Geometry check sheet. Reference: the model listing, model coordinates, mm. A direction names the side the tool comes from. Coordinates: 2 decimals unless noted, no trailing zeros. Order: outer loops, then holes, each group sorted by start corner. A loop starts at its lowest first (then second) coordinate and runs counter-clockwise, first axis right, second up. Notation, with made-up numbers: M 38.5,89.5 L 95.5,89.5 A16 ccw 95.5,106.5 Z; hole C 44,57.5 d5. An arc over 180 degrees is marked long. One line per item, written item: value. Start each with the question number.
1) Draft check along Y on faces 1 (the flat face through (-51, 76.2, 13)), 2 (the flat face through (-38.1, 0, 13)), 3 (the flat face through (-2, 14, 0)), 4 (the flat face through (36.512, 0, 13)). Enter one of: pulls with the +Y half, pulls with the -Y half, needs draft (parallel to the pull), parting line crosses it, or undercut.
2) Access from +Z, -Z, +X, -X, +Y, -Y to the whole of each face (thin tool, end or side, straight path). Record for faces 5 (the flat face through (141.288, 17, 13)), 6 (the flat face through (-141.288, 18, 13)), 7 (the flat face through (141.288, -18, 13)), 8 (the flat face through (38.1, 0, 13)).
3) Go/stop test with flat-tipped pins: P1, Ø8, axis at y = -14, z = 18, coming from the +X side; P2, Ø8, axis at y = 16, z = 17, coming from the -X side; P3, Ø2, axis at x = 81.5, z = 6.5, coming from the -Y side. Record where each tip stops, or that it passes through.
4) Thickness scan on L1, parallel to X at y = -6, z = 11.25 (1 decimal); L2, parallel to Y at x = 88, z = 10.5; L3, parallel to X at y = 62.5, z = 16.5. Record the ranges inside material, lowest first. Write a range as from..to.
5) Sectioned sample at B-B, the plane x = -116. Enter the section's corners in (y, z), then the cut area to 3 significant figures.
6) Sectioned sample at C-C, the plane y = 40. Enter the section's corners in (x, z).
7) Sectioned sample at A-A, the plane z = 13.75. State how many separate pieces and enclosed holes the cut face has, then the cut area to 3 significant figures.
```python
from build123d import *

# Parameters (mm, degrees)
F0_W     = 25.4
F0_H     = 50.8
F0_W_2   = 76.2
F0_W_3   = 1.5875
F0_H_2   = 19.05
F1_DEPTH = 25.4


with BuildPart() as f1:
    # F0 (on Top) → F1 (new body)
    with BuildSketch(Plane.XY):
        Polygon((63.5, 25.4), (38.1, 25.4), (38.1, 9.525), (38.1, -9.525), (38.1, -25.4), (63.5, -25.4), (88.9, -25.4), (88.9, 25.4), align=None)
        with Locations((50.8, 50.8)):
            Rectangle(F0_W, F0_H)
        with Locations((0, 50.8)):
            Rectangle(F0_W_2, F0_H)
        Polygon((-38.1, 9.525), (-38.1, 25.4), (-63.5, 25.4), (-88.9, 25.4), (-88.9, -25.4), (-63.5, -25.4), (-38.1, -25.4), (-38.1, -9.525), align=None)
        with Locations((-50.8, 50.8)):
            Rectangle(F0_W, F0_H)
        with Locations((0, 101.6)):
            Rectangle(F0_W_2, F0_H)
        with Locations((89.69375, 0)):
            Rectangle(F0_W_3, F0_H)
        with BuildLine():
            Line((-38.1, 127), (38.1, 127))
            Line((38.1, 127), (38.1, 139.7))
            ThreePointArc((38.1, 139.7), (34.3802561211, 148.6802561211), (25.4, 152.4))
            Line((25.4, 152.4), (-25.4, 152.4))
            ThreePointArc((-25.4, 152.4), (-34.3802561211, 148.6802561211), (-38.1, 139.7))
            Line((-38.1, 139.7), (-38.1, 127))
        make_face()
        with Locations((-89.69375, 0)):
            Rectangle(F0_W_3, F0_H)
        with Locations((0, -50.8)):
            Rectangle(F0_W_2, F0_H)
        with Locations((50.8, -50.8)):
            Rectangle(F0_W, F0_H)
        Polygon((141.2875, 25.4), (90.4875, 25.4), (90.4875, -25.4), (141.2875, -25.4), (141.2875, -9.525), (141.2875, 9.525), align=None)
        with Locations((-50.8, -50.8)):
            Rectangle(F0_W, F0_H)
        Polygon((-90.4875, -25.4), (-90.4875, 25.4), (-141.2875, 25.4), (-141.2875, 9.525), (-141.2875, -9.525), (-141.2875, -25.4), align=None)
        with Locations((142.08125, 0)):
            Rectangle(F0_W_3, F0_H_2)
        with Locations((-142.08125, 0)):
            Rectangle(F0_W_3, F0_H_2)
        Polygon((38.1, 9.525), (38.1, 25.4), (-38.1, 25.4), (-38.1, 9.525), (-36.5125, 9.525), (-36.5125, -9.525), (-38.1, -9.525), (-38.1, -25.4), (38.1, -25.4), (38.1, -9.525), (36.5125, -9.525), (36.5125, 9.525), align=None)
    extrude(amount=F1_DEPTH)


solid = f1.part
```
Final values:
1. face 1: pulls with the +Y half
1. face 2: undercut
1. face 3: needs draft
1. face 4: undercut
2. face 5: +Z, -Z, +X, +Y
2. face 6: +Z, -Z, -X, +Y
2. face 7: +Z, -Z, +X, -Y
2. face 8: +Z, -Z
3. P1: stops at x = 141.29
3. P2: stops at x = -141.29
3. P3: stops at y = -25.4
4. L1: x = -142.9..-38.1, -36.5..36.5, 38.1..142.9
4. L2: y = -25.4..25.4
4. L3: x = -63.5..63.5
5. outline: M -25.4,0 L 25.4,0 L 25.4,25.4 L -25.4,25.4 Z
5. area: 1,290 mm^2
6. outline: M -63.5,0 L 63.5,0 L 63.5,25.4 L -63.5,25.4 Z
7. separate pieces: 1
7. enclosed holes: 2
7. area: 33,000 mm^2
